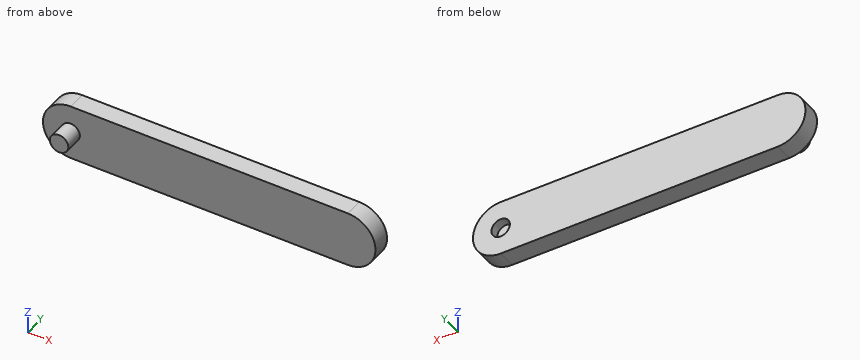
from build123d import *

# Parameters (mm, degrees)
BOSS_EXTRUDE1_DEPTH = 100
SKETCH3_R           = 50
BOSS_EXTRUDE3_DEPTH = 100
SKETCH2_R           = 50
CUT_EXTRUDE1_DEPTH  = 50


with BuildPart() as part:
    # Sketch1 → Boss-Extrude1 (new body)
    with BuildSketch(Plane(origin=(0, 0, 0), x_dir=(1, 0, 0), z_dir=(0, 1, 0))):
        with BuildLine():
            Line((0, 150), (1500, 150))
            ThreePointArc((1500, 150), (1650, 0), (1500, -150))
            Line((1500, -150), (0, -150))
            ThreePointArc((0, -150), (-150, 0), (0, 150))
        make_face()
    extrude(amount=BOSS_EXTRUDE1_DEPTH)

    # Sketch3 → Boss-Extrude3 (add)
    with BuildSketch(Plane.XZ):
        with Locations(Location((0, 0, 0), (0, 0, 90))):
            Circle(SKETCH3_R)
    extrude(amount=BOSS_EXTRUDE3_DEPTH)

    # Sketch2 → Cut-Extrude1 (cut)
    with BuildSketch(Plane(origin=(0, 100, 0), x_dir=(1, 0, 0), z_dir=(0, 1, 0))):
        with Locations(Location((1500, 0, 0), (0, 0, 270))):
            Circle(SKETCH2_R)
    extrude(amount=-CUT_EXTRUDE1_DEPTH, mode=Mode.SUBTRACT)


solid = part.part
Source: CAD feature listing. Evaluate the final solid. Frame: model axes, mm. Give positions to 0.01 mm unless a question says otherwise; leave off trailing zeros. Order: outer loops, then holes, each group sorted by start corner. A loop starts at its lowest first (then second) coordinate and runs counter-clockwise, first axis right, second up. Notation, with made-up numbers: (5.5, -12) -> (42.5, -12) arc R26 ccw to (42.5, 4) -> close; hole circle Ø7 at (23, -25). An arc over 180 degrees is marked (long way). Write item = value, one per line.
Q1. Cut plane D-D, the plane x = 339.5. Output: boundary loops of the cut face in (y, z), and give its area (3 significant figures).
Data:
outline = (0, -150) -> (100, -150) -> (100, 150) -> (0, 150) -> close
area = 30,000 mm^2
Q2. Material intervals for line 1 (X direction, y = 67, z = 0); line 2 (Y direction, x = 1096.5, z = 55); line 3 (X direction, y = 39.5, z = 112), sorted ascending. Write a range as from..to.
Data:
line_1 = -150..1450, 1550..1650
line_2 = 0..100
line_3 = -99.78..1599.78
Q3. Cut plane B-B, the plane x = -35. Output: boundary loops of the cut face in (y, z).
Data:
outline = (-100, -35.71) -> (0, -35.71) -> (0, -145.86) -> (100, -145.86) -> (100, 145.86) -> (0, 145.86) -> (0, 35.71) -> (-100, 35.71) -> close
Q4. Cut plane A-A, the plane z = 0. Output: boundary loops of the cut face in (x, y), and give its area (3 significant figures).
Data:
outline = (-150, 0) -> (-50, 0) -> (-50, -100) -> (50, -100) -> (50, 0) -> (1650, 0) -> (1650, 100) -> (1550, 100) -> (1550, 50) -> (1450, 50) -> (1450, 100) -> (-150, 100) -> close
area = 185,000 mm^2
Q5. Pin query (flat end, axial travel): pin 1 (1 mm diameter, centred on y = -18, z = 32.5, fed in from -X); pin 2 (12 mm diameter, centred on y = 12, z = 100.5, fed in from +X); pin 3 (6 mm diameter, centred on x = 170, z = 117.5, fed in from -Y). Return the tip coordinate at first contact, or that it passes through.
Data:
pin_1 = -38.42
pin_2 = 1616.49
pin_3 = 0
Q6. Cut plane C-C, the plane y = -33. Output: boundary loops of the cut face in (x, z).
Data:
outline = circle Ø100 at (0, 0)
